Build history of the part. All positions in model axes, mm. A direction names the side the tool comes from. Round coordinates to 2 decimals unless told otherwise and drop trailing zeros. Loops run counter-clockwise (first coordinate to the right, second up) from the corner with the lowest first, then second, coordinate; pieces in that order, holes last. Notation, with made-up numbers: (55, 60.5) -> (107, 60.5) arc R18 cw to (107, 78.5) -> close; hole circle Ø4 at (32, 15). An arc over 180 degrees is marked (long way). Put each result on its own line as item: value. Start each with the question number.
```python
from build123d import *

# Parameters (mm, degrees)
EXTRUSION_PROFILE_DEPTH                      = 303.2125
SKETCH3_R                                    = 1.7272
THRU_HOLES_FOR_DRIVER_ENCLOSURE_DEPTH        = 27.9875
WIRE_ROUTING_SLOT_DEPTH                      = 27.9875
SKETCH5_R                                    = 1.0922
F_4_40_TAPPED_HOLES_FOR_MAGNETIC_CATCH_DEPTH = 27.9875
F_1_4_20_TAPPED_HOLE_FOR_MOUNTING_BRACKET_D  = 5.1054
SKETCH9_R                                    = 1.0922
F_4_40_TAPPED_HOLES_FOR_LED_BOARD_DEPTH      = 27.9875


with BuildPart() as part:
    # Sketch1 → Extrusion Profile (new body, symmetric)
    with BuildSketch(Plane.XY):
        Polygon((-25.4, -25.4), (-25.4, 25.4), (-22.225, 25.4), (-22.225, 1.5875), (22.225, 1.5875), (22.225, 25.4), (25.4, 25.4), (25.4, -25.4), (22.225, -25.4), (22.225, -1.5875), (-22.225, -1.5875), (-22.225, -25.4), align=None)
    extrude(amount=EXTRUSION_PROFILE_DEPTH, both=True)

    # Sketch3 → Thru Holes for Driver Enclosure (cut, through all)
    with BuildSketch(Plane(origin=(0, 1.5875, 0), x_dir=(1, 0, 0), z_dir=(0, 1, 0))):
        with Locations((10.16, -58.547)):
            Circle(SKETCH3_R)
        with Locations((-10.16, 58.547)):
            Circle(SKETCH3_R)
    extrude(amount=-THRU_HOLES_FOR_DRIVER_ENCLOSURE_DEPTH, mode=Mode.SUBTRACT)

    # Sketch4 → Wire Routing Slot (cut, through all)
    with BuildSketch(Plane.XZ.offset(1.5875)):
        with BuildLine():
            Line((-11.27125, -33.3375), (-11.27125, -17.4625))
            ThreePointArc((-11.27125, -17.4625), (-8.89, -15.08125), (-6.50875, -17.4625))
            Line((-6.50875, -17.4625), (-6.50875, -33.3375))
            ThreePointArc((-6.50875, -33.3375), (-8.89, -35.71875), (-11.27125, -33.3375))
        make_face()
    extrude(amount=-WIRE_ROUTING_SLOT_DEPTH, mode=Mode.SUBTRACT)

    # Sketch5 → 4-40 Tapped Holes for Magnetic Catch (cut, through all)
    with BuildSketch(Plane(origin=(0, 1.5875, 0), x_dir=(1, 0, 0), z_dir=(0, 1, 0))):
        with Locations((-9.525, -288.544)):
            Circle(SKETCH5_R)
        with Locations((9.525, -288.544)):
            Circle(SKETCH5_R)
        with Locations((9.525, 288.544)):
            Circle(SKETCH5_R)
        with Locations((-9.525, 288.544)):
            Circle(SKETCH5_R)
    extrude(amount=-F_4_40_TAPPED_HOLES_FOR_MAGNETIC_CATCH_DEPTH, mode=Mode.SUBTRACT)

    # 1/4-20 Tapped Hole for Mounting Bracket (through all)
    with Locations(Plane(origin=(0, 1.5875, 0), x_dir=(1, 0, 0), z_dir=(0, 1, 0))):
        with Locations((0, -282.575)):
            f_1_4_20_tapped_hole_for_mounting_bracket = Hole(F_1_4_20_TAPPED_HOLE_FOR_MOUNTING_BRACKET_D / 2)

    # Mirror1: 1/4-20 Tapped Hole for Mounting Bracket across plane
    add(f_1_4_20_tapped_hole_for_mounting_bracket.mirror(Plane.XY), mode=Mode.SUBTRACT)

    # Sketch9 → 4-40 Tapped Holes for LED Board (cut, through all)
    with BuildSketch(Plane.XZ.offset(1.5875)):
        with Locations((0, -228.6)):
            Circle(SKETCH9_R)
        with Locations((0, -146.05)):
            Circle(SKETCH9_R)
        with Locations((0, 146.05)):
            Circle(SKETCH9_R)
        with Locations((0, 228.6)):
            Circle(SKETCH9_R)
    extrude(amount=-F_4_40_TAPPED_HOLES_FOR_LED_BOARD_DEPTH, mode=Mode.SUBTRACT)


solid = part.part
```
Item 1: Drop flat-ended pins along their axis: pin 1 (12 mm diameter, centred on x = -3, z = -109, fed in from -Y); pin 2 (6 mm diameter, centred on x = 14.5, z = -118, fed in from +Y). Give the stop position or say it passes through.
Item 2: Cut at A-A on y = 16. Write the cut outline in (x, z) (1 decimal), then the cut area to 3 significant figures.
Item 3: Cut at B-B on z = -217. Write the cut outline in (x, y) (1 decimal).
Item 4: Pull direction X, two halves, no side cores. Call faces 4 (the face through (0, 1.588, 4)), 5 (the face through (0, 0, -303.212)), 6 (the face through (25.4, 0, 4)): +X half, -X half, draft (parallel to the pull), parting line (faces both ways), or undercut.
Item 5: Wall check: line 1 (X direction, y = -7.5, z = 191) (3 decimals); line 2 (X direction, y = -0.8, z = 228.6); line 3 (Y direction, x = -5, z = -1.5). Give the ranges that are in metal, low to high. Write a range as from..to.
Item 6: 3-axis set-ups, long thin cutter, end or side, ignore diameter. For faces 1 (the face through (22.225, 13, 4)), 2 (the face through (0, -1.588, 4)), 3 (the face through (0, 0, 303.212)): which of +Z, -Z, +X, -X, +Y, -Y reach the whole face in a straight line?
Ans:
1. pin 1: stops at y = -1.59
1. pin 2: stops at y = 1.59
2. outline: (-25.4, -303.2) -> (-22.2, -303.2) -> (-22.2, 303.2) -> (-25.4, 303.2) -> close; (22.2, -303.2) -> (25.4, -303.2) -> (25.4, 303.2) -> (22.2, 303.2) -> close
2. area: 3,850 mm2
3. outline: (-25.4, -25.4) -> (-22.2, -25.4) -> (-22.2, -1.6) -> (22.2, -1.6) -> (22.2, -25.4) -> (25.4, -25.4) -> (25.4, 25.4) -> (22.2, 25.4) -> (22.2, 1.6) -> (-22.2, 1.6) -> (-22.2, 25.4) -> (-25.4, 25.4) -> close
4. face 4: undercut
4. face 5: draft
4. face 6: +X half
5. line 1: x = -25.4..-22.225, 22.225..25.4
5. line 2: x = -25.4..-1.09, 1.09..25.4
5. line 3: y = -1.59..1.59
6. face 1: +Z, -Z, +Y
6. face 2: +Z, -Z, -Y
6. face 3: +Z, +X, -X, +Y, -Y
